from build123d import *

# Parameters (mm, degrees)
CHAMFER_1_SIZE      = 1
SKETCH_2_W          = 5.515970317
SKETCH_2_H          = 8
CUT_EXTRUDE_1_DEPTH = 28
FILLET_1_R          = 4
FILLET_2_R          = 4


with BuildPart() as part:
    # 草图1 → 旋转1 (revolve)
    with BuildSketch(Plane.XY, mode=Mode.PRIVATE) as revolve_1_sk:
        Polygon((0, 0), (0, 10), (12, 10), (12, 8), (14, 8), (14, 12.5), (19, 12.5), (19, 20), (24, 20), (24, 12.5), (26, 12.5), (26, 14.5), (59, 14.5), (59, 11.5), (61, 11.5), (61, 12), (69, 12), (69, 11.5), (104, 11.5), (104, 8), (106, 8), (106, 10), (118, 10), (118, 0), align=None)
    revolve(revolve_1_sk.sketch.rotate(Axis((0, 0, 0), (-1, 0, 0)), 90), axis=Axis((0, 0, 0), (-1, 0, 0)))

    # 倒角1
    chamfer_1_edges = [part.edges().sort_by_distance(p)[0] for p in [
        (118, 0, 10),
        (59, 0, 14.5),
        (0, 0, 10),
    ]]
    chamfer(chamfer_1_edges, length=CHAMFER_1_SIZE)

    # 草图2 → 切除-拉伸1 (cut)
    with BuildSketch(Plane(origin=(29, 0, 0), x_dir=(0, 0, -1), z_dir=(1, 0, 0))):
        with Locations((-13.257985159, 0)):
            Rectangle(SKETCH_2_W, SKETCH_2_H)
    extrude(amount=CUT_EXTRUDE_1_DEPTH, mode=Mode.SUBTRACT)

    # 圆角1
    fillet_1_edges = [part.edges().sort_by_distance(p)[0] for p in [
        (29, 4, 12.218679932),
        (29, -4, 12.218679932),
    ]]
    fillet(fillet_1_edges, radius=FILLET_1_R - 0.0001)  # a hair under: the kernel refuses the full size

    # 圆角2
    fillet_2_edges = [part.edges().sort_by_distance(p)[0] for p in [
        (57, -4, 12.218679932),
        (57, 4, 12.218679932),
    ]]
    fillet(fillet_2_edges, radius=FILLET_2_R - 0.0001)  # a hair under: the kernel refuses the full size


solid = part.part
Can you work these out from the model? Positions are in its coordinate system, mm. A direction names the side the tool comes from. Coordinates: 2 decimals unless noted, no trailing zeros. Loops run counter-clockwise (first coordinate to the right, second up) from the corner with the lowest first, then second, coordinate; pieces in that order, holes last. Notation, with made-up numbers: M 13,68 L 42,68 A17 cw 42,80 Z; hole C -22.75,89 d9. An arc over 180 degrees is marked long. Return JSON: item names as keys, results as strings. Group by question number.
Item 1: Imagine slicing it at B-B (x = 95). Please give me the cut outline in (y, z), and give its area (3 significant figures).
Item 2: If I drill on L1, parallel to X at y = 6, z = 6; L2, parallel to X at y = -5, z = -11.5; L3, parallel to X at y = 11, z = 8.5, over which ranges is the centre line in solid material (lowest first)? Write a range as from..to.
Item 3: Imagine slicing it at A-A (x = 27.5). Please give me the cut outline in (y, z), and give its area (3 significant figures).
Item 4: I'm going to push flat-ended pins straight in: pin 1 Ø6.5 at (x, y) = (46, 1.5) entering from +Z; pin 2 Ø4 at (x, z) = (39.5, 13) entering from +Y; pin 3 Ø3 at (x, z) = (101, -3) entering from -Y. Where does each tip first touch, or does it pass through?
Item 5: On a 3-axis mill with a long thin cutter (end or side, diameter ignored), from which of +Z, -Z, +X, -X, +Y, -Y can I reach the whole of each face in a straight line? I mean faces 1 (the cylindrical face through (65.056, -3.604, -11.446)), 2 (the flat face through (43, 4, 12)), 3 (the flat face through (24, -9, -9)), 4 (the cylindrical face through (16.535, -3.755, -11.923)). Say none if no direction works.
Verdict:
{
 "1": {"outline": "C 0,0 d23", "area": "415 mm^2"},
 "2": {"L1": "x = 0..12, 14..104, 106..118", "L2": "x = 19..24, 26..59", "L3": "x = 19..24, 26..58.6"},
 "3": {"outline": "C 0,0 d29", "area": "661 mm^2"},
 "4": {"pin 1": "stops at z = 13.94", "pin 2": "stops at y = 9.45", "pin 3": "stops at y = -11.4"},
 "5": {"face 1": "+X", "face 2": "+Z", "face 3": "none", "face 4": "-X"}
}
